Input: part model. Units: mm. Frame: model coordinates. Round coordinates to 2 decimals unless told otherwise and drop trailing zeros. Loops run counter-clockwise (first coordinate to the right, second up) from the corner with the lowest first, then second, coordinate; pieces in that order, holes last. Notation, with made-up numbers: (67, 13.25) - (98, 13.25) arc R17 cw to (98, 25.25) - close; hole circle Ø1 at (-8.75, 36). An arc over 180 degrees is marked (long way). Write each question's results on one line, items separated by ' | '.
Autodesk Inventor part; units mm, degrees
ref_plane "YZ Plane" through (0, 0, 0) normal (1, 0, 0) x (0, 1, 0)
ref_plane "XZ Plane" through (0, 0, 0) normal (0, 1, 0) x (-1, 0, 0)
ref_plane "XY Plane" through (0, 0, 0) normal (0, 0, 1) x (1, 0, 0)
sketch "Boceto1" plane through (0, 0, 0) normal (0, 1, 0) x (-1, 0, 0)
  line L0 (0, 0) -> (13, 0)
  line L1 (13, 0) -> (13, -1.6)
  line L2 (13, -1.6) -> (0, -1.6)
  line L3 (0, -1.6) -> (0, 0)
  dimension "d0" = 13
  dimension "d1" = 1.6
extrude "Extrusión1" add sketch "Boceto1" along normal blind 10.06
sketch "Boceto3" plane through (0, 0, -1.6) normal (0, 0, -1) x (-1, 0, 0)
  circle A0 centre (2.25, 4) radius 0.5
  circle A1 centre (10.75, 4) radius 0.5
  line L0 (0, 0) -> (13, 0)
  dimension "d12" = 1
  dimension "d13" = 1
  dimension "d21" = 4
hole "Agujero1" at (-2.25, 4, -1.6) at (-10.75, 4, -1.6) at (-10.75, 4, -1.6) direction (0, 0, 1) diameter 1 end through all
properties part number "Placa Cobre" material "Cobre"
1. Section query A-A, the plane x = -10.75. Output: boundary loops of the cut face in (y, z).
Answer:
outline: (0, -1.6) - (3.5, -1.6) - (3.5, 0) - (0, 0) - close; (4.5, -1.6) - (10.06, -1.6) - (10.06, 0) - (4.5, 0) - close
2. Mould query, pull axis Y, two halves, no side actions, for faces 1 (the cylindrical face through (-10.262, 3.892, -0.789)), 2 (the flat face through (-13, 5, -1)), 3 (the flat face through (-6, 0, -1)), 4 (the flat face through (-6, 10.06, -1)). Classes: pulls with the +Y half, pulls with the -Y half, needs draft (parallel to the pull), parting line crosses it, or undercut.
Answer:
face 1: undercut | face 2: needs draft | face 3: pulls with the -Y half | face 4: pulls with the +Y half
3. Line query: line 1 (X direction, y = 4, z = -1.1); line 2 (Y direction, x = -10.75, z = -0.75). Output: solid intervals per line, ascending. Write a range as [from, to].
Answer:
line 1: [-13, -11.25], [-10.25, -2.75], [-1.75, 0] | line 2: [0, 3.5], [4.5, 10.06]
4. Section query B-B, the plane y = 4. Output: boundary loops of the cut face in (x, z), plus the area to 3 significant figures.
Answer:
outline: (-13, -1.6) - (-11.25, -1.6) - (-11.25, 0) - (-13, 0) - close; (-10.25, -1.6) - (-2.75, -1.6) - (-2.75, 0) - (-10.25, 0) - close; (-1.75, -1.6) - (0, -1.6) - (0, 0) - (-1.75, 0) - close | area: 17.6 mm^2
